Model file for the job. Use its own axes, mm. A direction names the side the tool comes from. Coordinates: 2 decimals unless noted, no trailing zeros. Order: outer loops, then holes, each group sorted by start corner. A loop starts at its lowest first (then second) coordinate and runs counter-clockwise, first axis right, second up.
from build123d import *

# Parameters (mm, degrees)
SKETCH_1_W                     = 80
SKETCH_1_H                     = 60
EXTRUDE_1_DEPTH                = 8
HOLE_WIZARD_M3_5_1_D           = 4
HOLE_WIZARD_M3_5_1_CBORE_D     = 8
HOLE_WIZARD_M3_5_1_CBORE_DEPTH = 2
SKETCH_14_W                    = 80
SKETCH_14_H                    = 2
SKETCH_14_W_2                  = 2
SKETCH_14_H_2                  = 16
CUT_EXTRUDE_1_DEPTH            = 1
CUT_EXTRUDE_2_REACH            = 92.174
SKETCH_15_R                    = 4.25
SKETCH_17_R                    = 11.5
CUT_EXTRUDE_4_DEPTH            = 4
SKETCH_18_R                    = 6
CUT_EXTRUDE_5_DEPTH            = 3
CHAMFER_1_SIZE                 = 1.499999999
CHAMFER_1_SIZE2                = 1.500000001
CHAMFER_2_SIZE                 = 1
SKETCH_20_W                    = 80
SKETCH_20_H                    = 6
CUT_EXTRUDE_6_DEPTH            = 1
SKETCH_21_W                    = 80
SKETCH_21_H                    = 4
CUT_EXTRUDE_7_DEPTH            = 1
SKETCH_22_W                    = 80
SKETCH_22_H                    = 2
CUT_EXTRUDE_8_DEPTH            = 1
SKETCH_23_R                    = 1
CUT_EXTRUDE_9_DEPTH            = 1
CUT_EXTRUDE_10_REACH           = 92.174
SKETCH_24_W                    = 80
SKETCH_24_H                    = 20


with BuildPart() as part:
    # 草图1 → 凸台-拉伸1 (new body)
    with BuildSketch(Plane.XY.offset(8)):
        with Locations((40, 10.833333333)):
            Rectangle(SKETCH_1_W, SKETCH_1_H)
    extrude(amount=-EXTRUDE_1_DEPTH)

    # M3.5 六角头机械螺钉的柱形沉头孔1 (through all)
    with Locations(Plane.XY.offset(8)):
        with Locations((8, 15.833333333), (72, 15.833333333)):
            CounterBoreHole(HOLE_WIZARD_M3_5_1_D / 2, HOLE_WIZARD_M3_5_1_CBORE_D / 2, HOLE_WIZARD_M3_5_1_CBORE_DEPTH)

    # 草图14 → 切除-拉伸1 (cut)
    with BuildSketch(Plane.XY.offset(8)):
        with Locations((40, 37.833333333)):
            Rectangle(SKETCH_14_W, SKETCH_14_H)
        Polygon((15, 40.833333333), (31, 24.833333333), (32.414213562, 26.247546896), (16.414213562, 42.247546896), align=None)
        with Locations((7, 32.833333333)):
            Rectangle(SKETCH_14_W_2, SKETCH_14_H_2)
        with Locations((40, 32.833333333)):
            Rectangle(SKETCH_14_W_2, SKETCH_14_H_2)
        with Locations((73, 32.833333333)):
            Rectangle(SKETCH_14_W_2, SKETCH_14_H_2)
        Polygon((47.585786438, 26.247546896), (63.585786438, 42.247546896), (65, 40.833333333), (49, 24.833333333), align=None)
    extrude(amount=-CUT_EXTRUDE_1_DEPTH, mode=Mode.SUBTRACT)

    # 草图15 → 切除-拉伸2 (cut, up to next)
    with BuildSketch(Plane.XY.offset(8), mode=Mode.PRIVATE) as cut_extrude_2_sk1:
        with Locations((40, 15.833333333)):
            Circle(SKETCH_15_R)
    cut_extrude_2_tool1 = extrude(cut_extrude_2_sk1.sketch, amount=-CUT_EXTRUDE_2_REACH, mode=Mode.PRIVATE) & part.part
    add(cut_extrude_2_tool1.solids().sort_by_distance((40, 15.833333, 8))[0], mode=Mode.SUBTRACT)

    # 草图17 → 切除-拉伸4 (cut)
    with BuildSketch(Plane.XY.offset(8)):
        with Locations((40, 15.833333333)):
            Circle(SKETCH_17_R)
    extrude(amount=-CUT_EXTRUDE_4_DEPTH, mode=Mode.SUBTRACT)

    # 草图18 → 切除-拉伸5 (cut)
    with BuildSketch(Plane(origin=(0, 0, 0), x_dir=(-1, 0, 0), z_dir=(0, 0, -1))):
        with Locations((-40, 15.833333333)):
            Circle(SKETCH_18_R)
    extrude(amount=-CUT_EXTRUDE_5_DEPTH, mode=Mode.SUBTRACT)

    # 倒角1
    chamfer_1_edges = [part.edges().sort_by_distance(p)[0] for p in [
        (74, 15.833333333, 0),
        (10, 15.833333333, 0),
    ]]
    chamfer_1_side = [part.faces().sort_by_distance(p)[0] for p in [
        (79, 10.833333333, 0),
    ]]
    chamfer(chamfer_1_edges, length=CHAMFER_1_SIZE, length2=CHAMFER_1_SIZE2, reference=chamfer_1_side[0])

    # 倒角2
    chamfer_2_edges = [part.edges().sort_by_distance(p)[0] for p in [
        (40, 40.833333333, 0),
    ]]
    chamfer(chamfer_2_edges, length=CHAMFER_2_SIZE)

    # 草图20 → 切除-拉伸6 (cut)
    with BuildSketch(Plane.XY.offset(8)):
        with Locations((40, -16.166666667)):
            Rectangle(SKETCH_20_W, SKETCH_20_H)
    extrude(amount=-CUT_EXTRUDE_6_DEPTH, mode=Mode.SUBTRACT)

    # 草图21 → 切除-拉伸7 (cut)
    with BuildSketch(Plane.XY.offset(7)):
        with Locations((40, -17.166666667)):
            Rectangle(SKETCH_21_W, SKETCH_21_H)
    extrude(amount=-CUT_EXTRUDE_7_DEPTH, mode=Mode.SUBTRACT)

    # 草图22 → 切除-拉伸8 (cut)
    with BuildSketch(Plane.XY.offset(6)):
        with Locations((40, -18.166666667)):
            Rectangle(SKETCH_22_W, SKETCH_22_H)
    extrude(amount=-CUT_EXTRUDE_8_DEPTH, mode=Mode.SUBTRACT)

    # 草图23 → 切除-拉伸9 (cut)
    with BuildSketch(Plane.XY.offset(8)):
        with Locations((7, 24.833333333)):
            Circle(SKETCH_23_R)
        with Locations((31.707106781, 25.540440115)):
            Circle(SKETCH_23_R)
        with Locations((48.292893219, 25.540440115)):
            Circle(SKETCH_23_R)
        with Locations((73, 24.833333333)):
            Circle(SKETCH_23_R)
    extrude(amount=-CUT_EXTRUDE_9_DEPTH, mode=Mode.SUBTRACT)

    # 草图24 → 切除-拉伸10 (cut, up to next)
    with BuildSketch(Plane.XY.offset(8), mode=Mode.PRIVATE) as cut_extrude_10_sk1:
        with Locations((40, -9.166666667)):
            Rectangle(SKETCH_24_W, SKETCH_24_H)
    cut_extrude_10_tool1 = extrude(cut_extrude_10_sk1.sketch, amount=-CUT_EXTRUDE_10_REACH, mode=Mode.PRIVATE) & part.part
    add(cut_extrude_10_tool1.solids().sort_by_distance((40, -9.166667, 8))[0], mode=Mode.SUBTRACT)


solid = part.part
Q1. Drop flat-ended pins along their axis: P1, Ø4, axis at x = 6.5, y = 16.5, coming from the +Z side; P2, Ø8, axis at x = 47.5, y = 20, coming from the -Z side; P3, Ø5, axis at x = 8, y = 15.83, coming from the -Z side. Give the stop position or say it passes through.
Established:
P1: stops at z = 6
P2: stops at z = 0
P3: stops at z = 1
Q2. Mould opens along Y. For faces 4 (the face through (52.805, 31.466, 7.507)), 5 (the face through (3, 40, 8)) say: pulls with the +Y half, pulls with the -Y half, needs draft (parallel to the pull), parting line crosses it, or undercut.
Established:
face 4: undercut
face 5: needs draft
Q3. Which spindle directions (+Z, -Z, +X, -X, +Y, -Y) get a long thin tool onto all of the face, cutting with end or side? Do faces 1 (the face through (28, 40, 8)), 2 (the face through (75.695, 14.301, 7.014)), 3 (the face through (36, 13, 3)). Say none if no direction does.
Established:
face 1: +Z, +X, -X, +Y, -Y
face 2: +Z
face 3: -Z
Q4. Cut at A-A, the plane x = 40. List the corners of the cut face in (y, z), plus the area to 4 significant figures.
Established:
outline: (0.83, 0) - (9.83, 0) - (9.83, 3) - (11.58, 3) - (11.58, 4) - (4.33, 4) - (4.33, 8) - (0.83, 8) - close; (20.08, 3) - (21.83, 3) - (21.83, 0) - (39.83, 0) - (40.83, 1) - (40.83, 7) - (27.33, 7) - (27.33, 4) - (20.08, 4) - close
area: 169.5 mm2
Q5. Cut at D-D, the plane y = 31.5. List the corners of the cut face in (x, z), plus the area to 3 significant figures.
Established:
outline: (0, 0) - (80, 0) - (80, 8) - (74, 8) - (74, 7) - (72, 7) - (72, 8) - (55.67, 8) - (55.67, 7) - (52.84, 7) - (52.84, 8) - (41, 8) - (41, 7) - (39, 7) - (39, 8) - (27.16, 8) - (27.16, 7) - (24.33, 7) - (24.33, 8) - (8, 8) - (8, 7) - (6, 7) - (6, 8) - (0, 8) - close
area: 628 mm2
Q6. Probe line 1 (Y direction, x = 8, z = 2.95); line 2 (Y direction, x = 3, z = 7.25); line 3 (Z direction, x = 34, y = 17). List the from-to ranges inside material, lowest first.
Established:
line 1: y = 0.83 to 13.83, 17.83 to 40.83
line 2: y = 0.83 to 36.83, 38.83 to 40.83
line 3: z = 0 to 4
Q7. Cut at C-C, the plane x = 24. List the corners of the cut face in (y, z), plus the area to 3 significant figures.
Established:
outline: (0.83, 0) - (39.83, 0) - (40.83, 1) - (40.83, 8) - (38.83, 8) - (38.83, 7) - (36.83, 7) - (36.83, 8) - (34.66, 8) - (34.66, 7) - (31.83, 7) - (31.83, 8) - (0.83, 8) - close
area: 315 mm2
Q8. Cut at B-B, the plane z = 2.25. List the corners of the cut face in (x, y), plus the area to 3 significant figures.
Established:
outline: (0, 0.83) - (80, 0.83) - (80, 40.83) - (0, 40.83) - close; hole circle Ø4 at (8, 15.83); hole circle Ø12 at (40, 15.83); hole circle Ø4 at (72, 15.83)
area: 3,060 mm2
